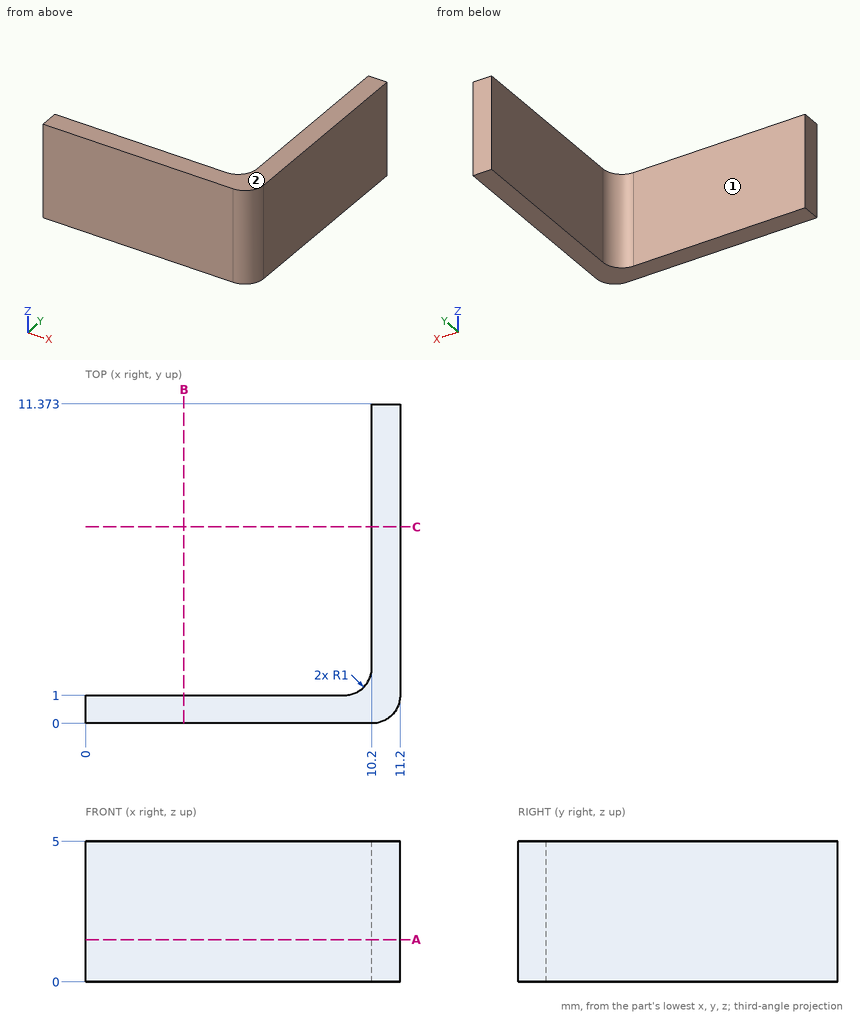
The drawing under review shows one solid part. Ordinate dimensions are in mm from its lowest x, y, z. A direction names the side the tool comes from. Round coordinates to 2 decimals unless told otherwise and drop trailing zeros. Loops run counter-clockwise (first coordinate to the right, second up) from the corner with the lowest first, then second, coordinate; pieces in that order, holes last. Notation, with made-up numbers: (79, 70.5) - (133, 70.5) arc R13 ccw to (133, 87.5) - close; hole circle Ø9 at (-13.5, 31). An arc over 180 degrees is marked (long way). Use a Markdown table: item, result. Add a question column.
Q1. Add section C-C (y = 7). State the section outline as (x, z) points.
Q2. Insertion check: pin 1 Ø3 at (y, z) = (4.5, 2.5) entering from -X; pin 2 Ø1.5 at (x, z) = (4, 2) entering from +Y. Each pin has a flat end and moves straight along its axis. Give the tip position at first contact, or say it passes through.
Q3. Add section A-A (z = 1.5). State the section outline as (x, y) points.
Q4. For probe 1 along X at (y, z) = (2.5, 1.95); probe 2 along Y at (x, z) = (6.75, 4); probe 3 along Y at (x, z) = (10.25, 3.3), list the stretches that pass through material, from the lowest coordinate up.
Q5. Add section B-B (x = 3.5). State the section outline as (y, z) points.
Q6. Machinability: for the marked faces 1 and 2, which of the approach directions +Z, -Z, +X, -X, +Y, -Y give a long, thin tool a straight path to every point of the face, cutting with its end or side? Answer none if there is none.
Worked answers:
| question | item | result |
|---|---|---|
| 1 | outline | (10.2, 0) - (11.2, 0) - (11.2, 5) - (10.2, 5) - close |
| 2 | pin 1 | x = 10.2 |
| 2 | pin 2 | y = 1 |
| 3 | outline | (0, 0) - (10.2, 0) arc R1 ccw to (11.2, 1) - (11.2, 11.37) - (10.2, 11.37) - (10.2, 2) arc R1 cw to (9.2, 1) - (0, 1) - close |
| 4 | probe 1 | 10.2 to 11.2 |
| 4 | probe 2 | 0 to 1 |
| 4 | probe 3 | 0 to 11.37 |
| 5 | outline | (0, 0) - (1, 0) - (1, 5) - (0, 5) - close |
| 6 | face 1 | +Z, -Z, -X, +Y |
| 6 | face 2 | +Z, +X, -X, +Y, -Y |
